from build123d import *

# Parameters (mm, degrees)
EXTRUDE_1_DEPTH     = 50
CUT_EXTRUDE_START   = -3.2
CUT_EXTRUDE_1_DEPTH = 43.6
SKETCH_1_4_R        = 6
SKETCH_1_4_R_2      = 3.5
CUT_EXTRUDE_2_DEPTH = 10
SKETCH_3_R          = 9.5
SKETCH_3_R_2        = 3.5
EXTRUDE_3_DEPTH     = 6
SKETCH_3_3_R        = 6.5
CUT_EXTRUDE_3_DEPTH = 3
SKETCH_3_4_R        = 7
CUT_EXTRUDE_4_DEPTH = 0.75


with BuildPart() as part:
    # Эскиз1 → Бобышка-Вытянуть1 (new body)
    with BuildSketch(Plane.XY):
        with BuildLine():
            Line((0, 0), (0, 5))
            Line((0, 5), (3, 5))
            ThreePointArc((3, 5), (7.242640687, 6.757359313), (9, 11))
            Line((9, 11), (9, 17.5))
            ThreePointArc((9, 17.5), (12.661165235, 26.338834765), (21.5, 30))
            Line((21.5, 30), (43.5, 30))
            ThreePointArc((43.5, 30), (52.338834765, 26.338834765), (56, 17.5))
            Line((56, 17.5), (56, 11))
            ThreePointArc((56, 11), (57.757359313, 6.757359313), (62, 5))
            Line((62, 5), (65, 5))
            Line((65, 5), (65, 0))
            Line((65, 0), (0, 0))
        make_face()
    extrude(amount=EXTRUDE_1_DEPTH)

    # Эскиз2 → Вырез-Вытянуть1 (cut)
    with BuildSketch(Plane(origin=(0, 0, 0), x_dir=(-1, 0, 0), z_dir=(0, 0, -1)).offset(CUT_EXTRUDE_START)):
        with BuildLine():
            Line((-21.5, 27.6), (-43.5, 27.6))
            ThreePointArc((-43.5, 27.6), (-50.64177849, 24.64177849), (-53.6, 17.5))
            Line((-53.6, 17.5), (-53.6, 0))
            Line((-53.6, 0), (-11.4, 0))
            Line((-11.4, 0), (-11.4, 17.5))
            ThreePointArc((-11.4, 17.5), (-14.35822151, 24.64177849), (-21.5, 27.6))
        make_face()
    extrude(amount=-CUT_EXTRUDE_1_DEPTH, mode=Mode.SUBTRACT)

    # Эскиз1<4> → Вырез-Вытянуть2 (cut)
    with BuildSketch(Plane.XY):
        with Locations((21.5, 17.5)):
            Circle(SKETCH_1_4_R)
        with Locations((43.5, 17.5)):
            Circle(SKETCH_1_4_R_2)
    extrude(amount=CUT_EXTRUDE_2_DEPTH, mode=Mode.SUBTRACT)

    # Эскиз3 → Бобышка-Вытянуть3 (add)
    with BuildSketch(Plane(origin=(0, 0, 0), x_dir=(-1, 0, 0), z_dir=(0, 0, -1))):
        with Locations((-43.5, 17.5)):
            Circle(SKETCH_3_R)
        with Locations((-43.5, 17.5)):
            Circle(SKETCH_3_R_2, mode=Mode.SUBTRACT)
    extrude(amount=-EXTRUDE_3_DEPTH)

    # Эскиз3<3> → Вырез-Вытянуть3 (cut)
    with BuildSketch(Plane(origin=(0, 0, 0), x_dir=(-1, 0, 0), z_dir=(0, 0, -1))):
        with Locations((-43.5, 17.5)):
            Circle(SKETCH_3_3_R)
    extrude(amount=-CUT_EXTRUDE_3_DEPTH, mode=Mode.SUBTRACT)

    # Эскиз3<4> → Вырез-Вытянуть4 (cut)
    with BuildSketch(Plane(origin=(0, 0, 0), x_dir=(-1, 0, 0), z_dir=(0, 0, -1))):
        with Locations((-21.5, 17.5)):
            Circle(SKETCH_3_4_R)
    extrude(amount=-CUT_EXTRUDE_4_DEPTH, mode=Mode.SUBTRACT)


solid = part.part
Can you work these out from the model? Positions are in its coordinate system, mm. A direction names the side the tool comes from. Coordinates: 2 decimals unless noted, no trailing zeros. Loops run counter-clockwise (first coordinate to the right, second up) from the corner with the lowest first, then second, coordinate; pieces in that order, holes last. Notation, with made-up numbers: (53, -20) - (107, -20) arc R32 cw to (107, 13) - close; hole circle Ø4 at (72.5, 41.25). An arc over 180 degrees is marked (long way). Put each result on its own line as item: value. Start each with the question number.
Item 1: If we mould it in two halves opening along Z, with no side actions, what happens to faces 6 (the face through (11.4, 9, 25)), 7 (the face through (16, 21, 0.75)), 8 (the face through (63, 5, 25))? For each: +Z half, -Z half, draft (parallel to the pull), parting line (faces both ways), or undercut.
Item 2: Suppose I cut it at D-D (x = 58.5). Please give me the cut outline in (y, z).
Item 3: Suppose I cut it at C-C (y = 15). Please give me the cut outline in (x, z), and give its area (3 significant figures).
Item 4: Suppose I cut it at B-B (z = 27). Please give me the cut outline in (x, y), and give its area (3 significant figures).
Item 5: Suppose I cut it at A-A (y = 20). Please give me the cut outline in (x, z), and give its area (3 significant figures).
Item 6: For pin 1 (5 mm diameter, centred on y = 14, z = 33, fed in from +X); pin 2 (5 mm diameter, centred on y = 12, z = 32, fed in from -X); pin 3 (1.5 mm diameter, centred on x = 25, y = 15, fed in from -Z), each with a flat end and sliding along its axis, tell me the tip position at first contact or that it passes through.
Item 7: If I drill on line 1 along Z through (x, y) = (20, 9.5); line 2 along X through (y, z) = (2, 10); line 3 along Z through (x, y) = (39, 11.5), over which ranges is the centre line in solid material (lowest first)?
Item 8: Which directions (+Z, -Z, +X, -X, +Y, -Y) give clear straight access to the entire face, cutting with the end or side of a thin tool? Please do faces 1 (the face through (1, 5, 25)), 2 (the face through (23.017, 10.666, 0.37)), 3 (the face through (33, 15, 50)), 4 (the face through (56, 14, 25)), 5 (the face through (53.6, 9, 25)).
Here are the results:
1. face 6: undercut
1. face 7: -Z half
1. face 8: draft
2. outline: (0, 0) - (6.13, 0) - (6.13, 50) - (0, 50) - close
3. outline: (9, 0) - (14.96, 0) - (14.96, 0.75) - (16.05, 0.75) - (16.05, 3.2) - (11.4, 3.2) - (11.4, 46.8) - (53.6, 46.8) - (53.6, 3.2) - (52.67, 3.2) - (52.67, 6) - (45.95, 6) - (45.95, 3) - (49.5, 3) - (49.5, 0) - (56, 0) - (56, 50) - (9, 50) - close; (26.95, 0.75) - (28.04, 0.75) - (28.04, 0) - (37.5, 0) - (37.5, 3) - (41.05, 3) - (41.05, 6) - (34.33, 6) - (34.33, 3.2) - (26.95, 3.2) - close
3. area: 474 mm²
4. outline: (0, 0) - (11.4, 0) - (11.4, 17.5) arc R10.1 cw to (21.5, 27.6) - (43.5, 27.6) arc R10.1 cw to (53.6, 17.5) - (53.6, 0) - (65, 0) - (65, 5) - (62, 5) arc R6 cw to (56, 11) - (56, 17.5) arc R12.5 ccw to (43.5, 30) - (21.5, 30) arc R12.5 ccw to (9, 17.5) - (9, 11) arc R6 cw to (3, 5) - (0, 5) - close
4. area: 327 mm²
5. outline: (9.25, 0) - (14.96, 0) - (14.96, 0.75) - (16.05, 0.75) - (16.05, 3.2) - (11.71, 3.2) - (11.71, 46.8) - (53.29, 46.8) - (53.29, 3.2) - (52.67, 3.2) - (52.67, 6) - (45.95, 6) - (45.95, 3) - (49.5, 3) - (49.5, 0) - (55.75, 0) - (55.75, 50) - (9.25, 50) - close; (26.95, 0.75) - (28.04, 0.75) - (28.04, 0) - (37.5, 0) - (37.5, 3) - (41.05, 3) - (41.05, 6) - (34.33, 6) - (34.33, 3.2) - (26.95, 3.2) - close
5. area: 476 mm²
6. pin 1: x = 56
6. pin 2: x = 8.81
6. pin 3: z = 46.8
7. line 1: 0 to 3.2, 46.8 to 50
7. line 2: 0 to 11.4, 53.6 to 65
7. line 3: 0 to 6, 46.8 to 50
8. face 1: +Z, -Z, -X, +Y
8. face 2: -Z
8. face 3: +Z, +X, -X, +Y, -Y
8. face 4: +Z, -Z, +X, +Y
8. face 5: -Y
